Source: CAD feature listing. Evaluate the final solid. Frame: model axes, mm. A direction names the side the tool comes from. Give positions to 0.01 mm unless a question says otherwise; leave off trailing zeros. Order: outer loops, then holes, each group sorted by start corner. A loop starts at its lowest first (then second) coordinate and runs counter-clockwise, first axis right, second up. Notation, with made-up numbers: M -30,40 L 3,40 A17 ccw 3,66 Z; hole C -10,49.25 d3. An arc over 180 degrees is marked long. Return JSON: item names as keys, results as strings.
Autodesk Inventor part; units mm, degrees
ref_plane "YZ Plane" through (0, 0, 0) normal (1, 0, 0) x (0, 1, 0)
ref_plane "XZ Plane" through (0, 0, 0) normal (0, 1, 0) x (-1, 0, 0)
ref_plane "XY Plane" through (0, 0, 0) normal (0, 0, 1) x (1, 0, 0)
sketch "Sketch1" plane through (0, 0, 0) normal (0, 0, 1) x (1, 0, 0)
  arc A0 (-3.85, 3.05) -> (-3.85, -3.95) centre (-3.85, -0.45) ccw
  arc A1 (-1.4191, -5) -> (-2.85, -3.95) centre (-2.85, -5.45) ccw
  line L0 (-2.85, -3.95) -> (-3.85, -3.95)
  arc A2 (-1.35, -5.45) -> (-1.4191, -5) centre (-2.85, -5.45) ccw
  line L1 (-1.35, -5.45) -> (-1.35, -6)
  line L2 (-1.35, -6) -> (-1.35, -14.05)
  line L3 (-1.35, -14.05) -> (-1.35, -15.05)
  line L4 (-1.35, -15.05) -> (-1.35, -22.75)
  arc A3 (-1.35, -22.75) -> (0.15, -24.25) centre (0.15, -22.75) ccw
  line L5 (0.15, -24.25) -> (2.6, -24.25)
  line L6 (24.3, -24.25) -> (2.6, -24.25)
  line L7 (24.3, -24.25) -> (26.75, -24.25)
  arc A4 (26.75, -24.25) -> (28.25, -22.75) centre (26.75, -22.75) ccw
  line L8 (28.25, -22.75) -> (28.25, -15.05)
  line L9 (28.25, -15.05) -> (28.25, -14.05)
  line L10 (28.25, -14.05) -> (28.25, -6)
  line L11 (28.25, -6) -> (28.25, -5.45)
  arc A5 (28.3191, -5) -> (28.25, -5.45) centre (29.75, -5.45) ccw
  arc A6 (29.75, -3.95) -> (28.3191, -5) centre (29.75, -5.45) ccw
  arc A7 (30.75, -3.95) -> (30.75, 3.05) centre (30.75, -0.45) ccw
  line L12 (30.75, -3.95) -> (29.75, -3.95)
  line L13 (29.75, 3.05) -> (30.75, 3.05)
  arc A8 (28.25, 4.55) -> (29.75, 3.05) centre (29.75, 4.55) ccw
  line L14 (28.25, 4.55) -> (28.25, 5)
  line L15 (28.25, 5) -> (28.25, 6)
  line L16 (28.25, 6) -> (28.25, 21.85)
  arc A9 (28.25, 21.85) -> (26.75, 23.35) centre (26.75, 21.85) ccw
  line L17 (25.45, 23.35) -> (26.55, 23.35)
  line L18 (26.75, 23.35) -> (26.55, 23.35)
  line L19 (0.35, 23.35) -> (0.15, 23.35)
  arc A10 (0.15, 23.35) -> (-1.35, 21.85) centre (0.15, 21.85) ccw
  line L20 (0.35, 23.35) -> (1.45, 23.35)
  line L21 (-1.35, 5) -> (-1.35, 21.15)
  line L22 (-1.35, 21.85) -> (-1.35, 21.15)
  line L23 (-1.35, 5) -> (-1.35, 4.55)
  arc A11 (-2.85, 3.05) -> (-1.35, 4.55) centre (-2.85, 4.55) ccw
  line L24 (-3.85, 3.05) -> (-2.85, 3.05)
  line L25 (1.45, 23.35) -> (25.45, 23.35)
  point P0 (0, 0)
extrude "Extrusion1" add sketch "Sketch1" along normal blind 9
ref_plane "Work Plane1" through (13.45, 4.55, 0) normal (-1, 0, 0) x (0, 0, 1)
sketch "Sketch2" plane through (13.45, 4.55, 0) normal (-1, 0, 0) x (0, 0, 1)
  line L0 (9, -8.5) -> (9, -1.5)
  circle A0 centre (36, 9.4) radius 30
  line L1 (9, 9.4) -> (36, 9.4)
  line L2 (36, 9.4) -> (66, 9.4)
  line L3 (9, 9.4) -> (6, 9.4)
  line L4 (-3, 9.8) -> (-3, 9)
  line L5 (9, -1.5) -> (9, -8.5)
  line L6 (9, -8.5) -> (9, -10)
  line L7 (9, -10) -> (9, -27.3)
  line L8 (9, -27.3) -> (9, -28.8)
  line L9 (9, -28.8) -> (9, -27.3)
  line L10 (9, -27.3) -> (9, -10)
  line L11 (9, -10) -> (9, -8.5)
  line L12 (9, -8.5) -> (9, -1.5)
  line L13 (9, -1.5) -> (9, 0)
  line L14 (9, 0) -> (9, 17.3)
  line L15 (9, 17.3) -> (9, 18.8)
  line L16 (9, 18.8) -> (9, 17.3)
  line L17 (9, 17.3) -> (9, 0)
  line L18 (9, 0) -> (9, -1.5)
  line L19 (9, 9.4) -> (-3, 9.4)
  point P0 (0, -4.55)
  dimension "d2" = 60
  dimension "d3" = 27
revolve "Revolution1" cut sketch "Sketch2" angle 360 about axis through (13.45, 13.95, 9) along (0, 0, 1) contours A0 L3 L14 L13 L0 | L0 L13 L14 L1 L2 A0
shell "Shell1" thickness 1 removed faces 1 at (9.0167, -11.7167, 0)
sketch "Sketch4" plane through (26.75, 22.35, 8) normal (0, 0, -1) x (-1, 0, 0)
  arc A0 (2.983, 0) -> (23.617, 0) centre (13.3, -8.4) ccw
  arc A1 (30.6, -25.3) -> (30.6, -20.3) centre (30.6, -22.8) ccw
  line L0 (29.6, -20.3) -> (30.6, -20.3)
  arc A2 (27.1, -17.8) -> (29.6, -20.3) centre (29.6, -17.8) ccw
  line L1 (27.1, -0.5) -> (27.1, -17.8)
  arc A3 (27.1, -0.5) -> (26.6, 0) centre (26.6, -0.5) ccw
  line L2 (23.617, 0) -> (26.6, 0)
  arc A4 (0, 0) -> (-0.5, -0.5) centre (0, -0.5) ccw
  line L3 (-0.5, -17.8) -> (-0.5, -0.5)
  arc A5 (-3, -20.3) -> (-0.5, -17.8) centre (-3, -17.8) ccw
  line L4 (-4, -20.3) -> (-3, -20.3)
  arc A6 (-4, -20.3) -> (-4, -25.3) centre (-4, -22.8) ccw
  line L5 (-3, -25.3) -> (-4, -25.3)
  arc A7 (-0.5, -27.8) -> (-3, -25.3) centre (-3, -27.8) ccw
  line L6 (-0.5, -45.1) -> (-0.5, -27.8)
  arc A8 (-0.5, -45.1) -> (0, -45.6) centre (0, -45.1) ccw
  line L7 (26.6, -45.6) -> (0, -45.6)
  arc A9 (26.6, -45.6) -> (27.1, -45.1) centre (26.6, -45.1) ccw
  line L8 (27.1, -27.8) -> (27.1, -45.1)
  arc A10 (29.6, -25.3) -> (27.1, -27.8) centre (29.6, -27.8) ccw
  line L9 (30.6, -25.3) -> (29.6, -25.3)
  line L10 (-0.5, -27.8) -> (-0.5, -17.8)
  line L11 (27.1, -27.8) -> (27.1, -17.8)
  line L12 (0, 0) -> (2.983, 0)
  point P0 (26.75, -22.35)
extrude "Extrusion2" add sketch "Sketch4" along normal up to surface (8 mm away) contours L10 A7 L5 A6 L4 A5 | A2 L0 A1 L9 A10 L11
sketch "Sketch5" plane through (0, 0, 0) normal (0, 0, -1) x (-1, 0, 0)
  circle A0 centre (-30.75, -0.45) radius 1.7
  circle A1 centre (3.85, -0.45) radius 1.7
  point P0 (0, 0)
hole "Hole1" at (30.75, -0.45, 0) at (-3.85, -0.45, 0) direction (0, 0, 1) diameter 2.459 end through all
sketch "Sketch6" plane through (0.15, -24.25, 0) normal (0, -1, 0) x (1, 0, 0)
  line L0 (0, 0) -> (26.6, 0)
  line L1 (26.6, 0) -> (26.6, 9)
  line L2 (0, 9) -> (26.6, 9)
  line L3 (0, 0) -> (0, 9)
  line L4 (2.45, -3) -> (2.45, 0)
  line L5 (24.15, -3) -> (24.15, 0)
  line L6 (2.45, 0) -> (24.15, 0)
  line L7 (24.15, 0) -> (24.15, 7)
  line L8 (24.15, 7) -> (2.45, 7)
  line L9 (2.45, 7) -> (2.45, 0)
  point P0 (-0.15, 0)
  dimension "d15" = 2
extrude "Extrusion3" cut sketch "Sketch6" against normal blind 9 contours L9 L8 L7 L0
properties part number "SphereMount"
1. Section query B-B (x = 18). Return loops of the section in (y, z), then the cut area to 3 significant figures.
Evaluation:
{"outline": "M -24.25,7 L -23.25,7 L -23.25,8 L 1.45,8 A30.66 ccw 22.35,6.51 L 22.35,0 L 23.35,0 L 23.35,7.88 A29.65 cw 1.69,9 L -24.25,9 Z", "area": "56.0 mm^2"}
2. Section query A-A (y = -0.45). Return loops of the section in (x, z), then the cut area to 3 significant figures.
Evaluation:
{"outline": "M -7.35,0 L -5.08,0 L -5.08,9 L -7.35,9 Z; M -2.62,0 L -0.35,0 L -0.35,8 L 27.25,8 L 27.25,0 L 29.52,0 L 29.52,9 L -2.62,9 Z; M 31.98,0 L 34.25,0 L 34.25,9 L 31.98,9 Z", "area": "109 mm^2"}
3. Section query C-C (z = 2). State how many separate pieces and enclosed holes the cut face has, then the cut area to 3 significant figures.
Evaluation:
{"separate pieces": "1", "enclosed holes": "2", "area": "193 mm^2"}
4. Set-up query: faces 1 (the face through (30, 3.05, 4)), 2 (the face through (14, -24, 7)), 3 (the face through (14, 22.35, 4)), 4 (the face through (-3.3, -3.95, 4.4)). Return all of +Z, -Z, +X, -X, +Y, -Y with unobstructed straight access to the full face (end or side cutting, diameter ignored); none if empty.
Evaluation:
{"face 1": "+Z, -Z, +X, +Y", "face 2": "-Z, -Y", "face 3": "-Z", "face 4": "+Z, -Z, -X, -Y"}
5. First-contact query: pin 1 (4 mm diameter, centred on x = 20, y = -18, fed in from -Z); pin 2 (2 mm diameter, centred on y = -7.5, z = 1.5, fed in from +X); pin 3 (4 mm diameter, centred on x = 12.5, y = 18, fed in from -Z). Flat tips, straight axial feed; report the tip coordinate or a pass-through.
Evaluation:
{"pin 1": "stops at z = 8", "pin 2": "stops at x = 28.25", "pin 3": "stops at z = 5.08"}
6. Ray query, probe 1 along X at (y, z) = (-0.45, 4.25); probe 2 along Y at (x, z) = (-3.85, 3.5); probe 3 along X at (y, z) = (12, 2.75). Return the intervals inside material, ascending.
Evaluation:
{"probe 1": "x = -7.35 to -5.08, -2.62 to -0.35, 27.25 to 29.52, 31.98 to 34.25", "probe 2": "y = -3.95 to -1.68, 0.78 to 3.05", "probe 3": "x = -1.35 to -0.35, 27.25 to 28.25"}
7. Section query D-D (y = -7.5). Return loops of the section in (x, z), then the cut area to 3 significant figures.
Evaluation:
{"outline": "M -1.35,0 L -0.35,0 L -0.35,8 L 27.25,8 L 27.25,0 L 28.25,0 L 28.25,9 L -1.35,9 Z", "area": "45.6 mm^2"}
8. Draft query along Y for faces 5 (the face through (27.25, -1, 4)), 6 (the face through (-3.4, 3.05, 4.4)), 7 (the face through (-1, 3, 0)). Return one class per face: pulls with the +Y half, pulls with the -Y half, needs draft (parallel to the pull), parting line crosses it, or undercut.
Evaluation:
{"face 5": "undercut", "face 6": "pulls with the +Y half", "face 7": "needs draft"}
